Check sheet for the modelled part. Datum: model origin and axes. Units: mm. A direction names the side the tool comes from. Round coordinates to 2 decimals unless told otherwise and drop trailing zeros. Loops run counter-clockwise (first coordinate to the right, second up) from the corner with the lowest first, then second, coordinate; pieces in that order, holes last. Notation, with made-up numbers: (66, 29.25) - (100, 29.25) arc R22 ccw to (100, 61.25) - close; hole circle Ø5 at (16, 34.5). An arc over 180 degrees is marked (long way). Put each result on its own line as item: value.
```python
from build123d import *

# Parameters (mm, degrees)
ESTRUSIONE_ESTRUSIONE2_DEPTH      = 3.6
ESTRUSIONE_ESTRUSIONE2_DEPTH_BACK = 36
SCHIZZO1_W                        = 110
SCHIZZO1_H                        = 160
SVUOTA3_T                         = -1
ESTRUSIONE_ESTRUSIONE3_REACH      = 106.475
SCHIZZO32_W                       = 110
SCHIZZO32_H                       = 1


with BuildPart() as part:
    # Schizzo1 → Estrusione-Estrusione2 (new, two sides: drawn at the far end of the back side and taken through both)
    with BuildSketch(Plane.XY.offset(-ESTRUSIONE_ESTRUSIONE2_DEPTH_BACK)):
        Rectangle(SCHIZZO1_W, SCHIZZO1_H)
    extrude(amount=ESTRUSIONE_ESTRUSIONE2_DEPTH + ESTRUSIONE_ESTRUSIONE2_DEPTH_BACK)

    # Svuota3
    svuota3_openings = [part.faces().sort_by_distance(p)[0] for p in [
        (0, 80, -16.2),
    ]]
    offset(amount=SVUOTA3_T, openings=svuota3_openings, kind=Kind.INTERSECTION)

    # Schizzo32 → Estrusione-Estrusione3 (add, up to next)
    with BuildSketch(Plane.XY.offset(-35), mode=Mode.PRIVATE) as estrusione_estrusione3_sk1:
        with Locations((0, 79.5)):
            Rectangle(SCHIZZO32_W, SCHIZZO32_H)
    estrusione_estrusione3_tool1 = extrude(estrusione_estrusione3_sk1.sketch, amount=ESTRUSIONE_ESTRUSIONE3_REACH, mode=Mode.PRIVATE) - part.part
    add(estrusione_estrusione3_tool1.solids().sort_by_distance((0, 79.5, -35))[0])


solid = part.part
```
Item 1: Tool access check on faces 1 (the flat face through (-55, -1, -16)), 2 (the flat face through (-1, 1, 2.6)). Record the directions out of +Z, -Z, +X, -X, +Y, -Y that give a thin tool (end or side, any length) a straight path to the whole face; none if there is none.
Filled sheet:
face 1: +Z, -Z, -X, +Y, -Y
face 2: none
Item 2: Section check B-B on x = -11. Enter the section's corners in (y, z), then the cut area to 3 significant figures.
Filled sheet:
outline: (-80, -36) - (80, -36) - (80, 3.6) - (-80, 3.6) - close; hole (-79, -35) - (79, -35) - (79, 2.6) - (-79, 2.6) - close
area: 395 mm²
Item 3: Release check for a two-part mould opening along Y. For faces 3 (the flat face through (-1, 1, 3.6)), 4 (the flat face through (-1, 80, -16)), 5 (the flat face through (-1, 1, -35)), 6 (the flat face through (-1, -80, -16)) record: +Y half, -Y half, draft (parallel to the pull), parting line (faces both ways), or undercut.
Filled sheet:
face 3: draft
face 4: +Y half
face 5: undercut
face 6: -Y half
Item 4: Thickness scan on line 1 (X direction, y = 32.5, z = -33); line 2 (Z direction, x = 15.5, y = 60); line 3 (Y direction, x = 41, z = -23.5). Record the ranges inside material, lowest first. Write a range as from..to.
Filled sheet:
line 1: -55..-54, 54..55
line 2: -36..-35, 2.6..3.6
line 3: -80..-79, 79..80
Item 5: Section check A-A on z = -19. Enter the section's corners in (x, y).
Filled sheet:
outline: (-55, -80) - (55, -80) - (55, 80) - (-55, 80) - close; hole (-54, -79) - (54, -79) - (54, 79) - (-54, 79) - close
